from build123d import *

# Parameters (mm, degrees)
MAINBASESKETCH_W          = 15.8
MAINBASESKETCH_H          = 3.2
MAINBASEEXTRUDE_DEPTH     = 7.9
STUDSSKETCH_R             = 2.4
STUDSEXTRUDE_DEPTH        = 1.6
STUDSPATTERN_COUNT        = 2
STUDSPATTERN_PITCH        = 8
MAINBASESHELL_T           = -1.2
UNDERSIDECIRCLEEXT_START  = -0.2
UNDERSIDECIRCLESKETCH_R   = 3.15
UNDERSIDECIRCLESKETCH_R_2 = 2.4
UNDERSIDECIRCLEEXT_DEPTH  = 1.6


with BuildPart() as part:
    # MainBaseSketch → MainBaseExtrude (new, symmetric)
    with BuildSketch(Plane.XY):
        with Locations((8.581967213, 1.6)):
            Rectangle(MAINBASESKETCH_W, MAINBASESKETCH_H)
    extrude(amount=MAINBASEEXTRUDE_DEPTH, both=True)

    # StudsSketch → StudsExtrude (add)
    with BuildSketch(Plane(origin=(0, 3.2, 0), x_dir=(1, 0, 0), z_dir=(0, 1, 0))):
        with Locations((4.581967213, 4)):
            Circle(STUDSSKETCH_R)
    studsextrude = extrude(amount=STUDSEXTRUDE_DEPTH)

    # StudsPattern: StudsExtrude ×2
    with Locations(*[(0, 0, i * STUDSPATTERN_PITCH) for i in range(1, STUDSPATTERN_COUNT)]):
        add(studsextrude)

    # MainBaseShell
    mainbaseshell_openings = [part.faces().sort_by_distance(p)[0] for p in [
        (8.581967213, 0, 0),
    ]]
    offset(amount=MAINBASESHELL_T, openings=mainbaseshell_openings, kind=Kind.INTERSECTION)

    # UnderSideCircleSketch → UnderSideCircleExt (add)
    with BuildSketch(Plane.XZ.offset(-2).offset(UNDERSIDECIRCLEEXT_START)):
        with Locations((8.581967213, 0)):
            Circle(UNDERSIDECIRCLESKETCH_R)
        with Locations((8.581967213, 0)):
            Circle(UNDERSIDECIRCLESKETCH_R_2, mode=Mode.SUBTRACT)
    extrude(amount=UNDERSIDECIRCLEEXT_DEPTH)


solid = part.part
Design review of the part built by this model. Coordinates are the model's own, in mm. A direction names the side the tool comes from. Give positions to 0.01 mm unless a question says otherwise; leave off trailing zeros. Loops run counter-clockwise (first coordinate to the right, second up) from the corner with the lowest first, then second, coordinate; pieces in that order, holes last. Notation, with made-up numbers: M 69,-9 L 99,-9 A24 ccw 99,26 Z; hole C -34,21.25 d10. An arc over 180 degrees is marked long. Answer as a JSON object with one key per item and string values.
Item 1: Machinability: for faces 1 (the face through (9.872, 1.31, 2.024)), 2 (the face through (8, 2, -7.9)), 3 (the face through (5.872, 3.989, -6.024)), which of the approach directions +Z, -Z, +X, -X, +Y, -Y give a long, thin tool a straight path to every point of the face, cutting with its end or side? Answer none if there is none.
Output values:
{"face 1": "-Y", "face 2": "-Z, +X, -X, +Y, -Y", "face 3": "+Y"}
Item 2: For P1, Ø1.9, axis at x = 4.5, z = -4.5, coming from the -Y side; P2, Ø1.5, axis at x = 10.5, z = 6, coming from the +Y side; P3, Ø0.7, axis at x = 4.5, z = 4.5, coming from the -Y side, all flat-tipped, find the tip position at first contact; note any pin that passes through.
Output values:
{"P1": "stops at y = 2", "P2": "stops at y = 3.2", "P3": "stops at y = 3.6"}
Item 3: We need section C-C (x = 2.75). State the section outline as (y, z) points, and give its area (3 significant figures).
Output values:
{"outline": "M 0,-7.9 L 3.2,-7.9 L 3.2,-5.55 L 4.8,-5.55 L 4.8,-2.45 L 3.2,-2.45 L 3.2,2.45 L 4.8,2.45 L 4.8,5.55 L 3.2,5.55 L 3.2,7.9 L 0,7.9 L 0,6.7 L 2,6.7 L 2,-6.7 L 0,-6.7 Z", "area": "33.7 mm2"}
Item 4: We need section B-B (z = -4). State the section outline as (x, y) points.
Output values:
{"outline": "M 0.68,0 L 1.88,0 L 1.88,2 L 3.38,2 L 3.38,3.6 L 5.78,3.6 L 5.78,2 L 15.28,2 L 15.28,0 L 16.48,0 L 16.48,3.2 L 6.98,3.2 L 6.98,4.8 L 2.18,4.8 L 2.18,3.2 L 0.68,3.2 Z"}
Item 5: We need section A-A (y = 1.1). State the section outline as (x, z) points.
Output values:
{"outline": "M 0.68,-7.9 L 16.48,-7.9 L 16.48,7.9 L 0.68,7.9 Z; C 8.58,0 d6.3; hole M 1.88,-6.7 L 15.28,-6.7 L 15.28,6.7 L 1.88,6.7 Z; hole C 8.58,0 d4.8"}
Item 6: Wall thickness on line 1 along X through (y, z) = (1.15, 0); line 2 along Z through (x, y) = (14.75, 0.9); line 3 along X through (y, z) = (0.55, 2): over which ranges is each line inside the solid? List them lowest first.
Output values:
{"line 1": "x = 0.68 to 1.88, 5.43 to 6.18, 10.98 to 11.73, 15.28 to 16.48", "line 2": "z = -7.9 to -6.7, 6.7 to 7.9", "line 3": "x = 0.68 to 1.88, 15.28 to 16.48"}
Item 7: We need section D-D (y = 3.4). State the section outline as (x, z) points.
Output values:
{"outline": "C 4.58,-4 d4.8; C 4.58,4 d4.8; hole C 4.58,-4 d2.4; hole C 4.58,4 d2.4"}
Item 8: Mouldability with a two-part tool opening along Z and no side actions: class faces 4 (the face through (8, 1, -6.7)), 5 (the face through (8, 2, 7.9)), 6 (the face through (16.482, 2, 0)) as pulls with the +Z half, pulls with the -Z half, needs draft (parallel to the pull), parting line crosses it, or undercut.
Output values:
{"face 4": "undercut", "face 5": "pulls with the +Z half", "face 6": "needs draft"}
